Can you work these out from the model? Positions are in its coordinate system, mm. Give positions to 0.01 mm unless a question says otherwise; leave off trailing zeros. Loops run counter-clockwise (first coordinate to the right, second up) from the corner with the lowest first, then second, coordinate; pieces in that order, holes last.
Autodesk Inventor part; units mm, degrees
ref_plane "YZ Plane" through (0, 0, 0) normal (1, 0, 0) x (0, 1, 0)
ref_plane "XZ Plane" through (0, 0, 0) normal (0, 1, 0) x (-1, 0, 0)
ref_plane "XY Plane" through (0, 0, 0) normal (0, 0, 1) x (1, 0, 0)
sketch "Sketch1" plane through (0, 0, 0) normal (0, 1, 0) x (-1, 0, 0)
  circle A0 centre (0, 0) radius 25 construction
  line L0 (25, -12.0394) -> (6.1745, -27.0522)
  line L1 (6.1745, -27.0522) -> (-17.3005, -21.6942)
  line L2 (-17.3005, -21.6942) -> (-27.7479, 0)
  line L3 (-27.7479, 0) -> (-17.3005, 21.6942)
  line L4 (-17.3005, 21.6942) -> (6.1745, 27.0522)
  line L5 (6.1745, 27.0522) -> (25, 12.0394)
  line L6 (25, 12.0394) -> (25, -12.0394)
  point P0 (25, 0)
  dimension "d0" = 50
extrude "Extrusion1" add sketch "Sketch1" along normal blind 4
properties part number "objeto6"
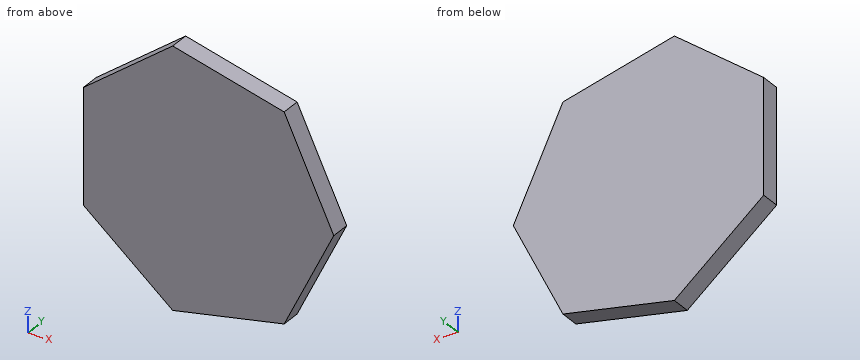
(1) Suppose I cut it at C-C on z = 7. List the corners of the cut face in (x, y) for me, plus the area to 3 significant figures.
Returned:
outline: (-25, 0) - (24.38, 0) - (24.38, 4) - (-25, 4) - close
area: 198 mm2
(2) Suppose I cut it at A-A on y = 0.7. List the corners of the cut face in (x, z) for me, plus the area to 3 significant figures.
Returned:
outline: (-25, -12.04) - (-6.17, -27.05) - (17.3, -21.69) - (27.75, 0) - (17.3, 21.69) - (-6.17, 27.05) - (-25, 12.04) - close
area: 2,110 mm2
(3) Please list where these lines run through material, in increasing order: probe 1 along X at (y, z) = (0.3, 7); probe 2 along X at (y, z) = (2.45, 7.5); probe 3 along Z at (x, y) = (21.5, 2.75).
Returned:
probe 1: x = -25 to 24.38
probe 2: x = -25 to 24.14
probe 3: z = -12.97 to 12.97
(4) Will this pin go through, and if not, where does the flat tip stop? P1, Ø12, axis at x = -6, z = 9, coming from the -Y side.
Returned:
P1: stops at y = 0
(5) Suppose I cut it at B-B on x = 13. List the corners of the cut face in (y, z) for me.
Returned:
outline: (0, -22.68) - (4, -22.68) - (4, 22.68) - (0, 22.68) - close
